Check sheet for the modelled part. Datum: model origin and axes. Units: mm. A direction names the side the tool comes from. Give positions to 0.01 mm unless a question says otherwise; leave off trailing zeros. Order: outer loops, then holes, each group sorted by start corner. A loop starts at its lowest first (then second) coordinate and runs counter-clockwise, first axis right, second up.
Item 1: Access from +Z, -Z, +X, -X, +Y, -Y to the whole of each face (thin tool, end or side, straight path). Record for faces 4 (the flat face through (0, 0, -14)), 5 (the flat face through (9.4, -2.9, 58.5)), 6 (the flat face through (0, -11.389, 62)), 7 (the flat face through (10, 0, 10)), 8 (the cylindrical face through (0, 14, 35)).
Item 2: Release check for a two-part mould opening along X. For faces 1 (the flat face through (0, -9, 59)), 2 (the cylindrical face through (3.233, 1.341, -0.986)), 3 (the cylindrical face through (11.5, 0.07, 4.93)) record: released by +X, released by -X, zero draft, split by the parting line, or undercut.
Item 3: Sectioned sample at A-A on z = 24. Record the boundary of the cut face in (x, y).
Item 4: Gauge pin test, flat ends, axial feed: P1, Ø1.5, axis at x = -9, y = -10, coming from the -Z side; P2, Ø4.5, axis at x = -2, y = -3.5, coming from the +Z side; P3, Ø1.5, axis at x = -10, y = 0, coming from the -Z side. Record the tip position at first contact, or that the pin passes through.
Item 5: Material ranges on line 1 along Z through (x, y) = (7.5, 6); line 2 along Y through (x, z) = (3.75, 42); line 3 along Z through (x, y) = (-10, -1), recorded low to high.
from build123d import *

# Parameters (mm, degrees)
SKETCH1_R            = 14
BOSS_EXTRUDE1_DEPTH  = 21
SKETCH2_R            = 13.5
BOSS_EXTRUDE2_DEPTH  = 0.5
SKETCH3_R            = 14
BOSS_EXTRUDE3_DEPTH  = 4
SKETCH4_R            = 14.5
BOSS_EXTRUDE4_DEPTH  = 20
SKETCH5_R            = 14
BOSS_EXTRUDE5_DEPTH  = 13
FILLET1_R            = 1
SKETCH6_R            = 14
SKETCH6_R_2          = 13.74791831
BOSS_EXTRUDE6_DEPTH  = 0.5
FILLET2_R            = 1
SKETCH7_R            = 5
BOSS_EXTRUDE7_DEPTH  = 3
SKETCH8_R            = 4.460837006
SKETCH8_R_2          = 1.021238478
CUT_EXTRUDE1_DEPTH   = 0.5
BOSS_EXTRUDE8_DEPTH  = 0.5
SKETCH10_W           = 3
SKETCH10_H           = 0.113026654
SKETCH10_H_2         = 0.277660136
BOSS_EXTRUDE9_DEPTH  = 6.5
FILLET3_R            = 0.4
CUT_EXTRUDE2_DEPTH   = 72.907798758
CUT_EXTRUDE3_DEPTH   = 0.1
CIRPATTERN1_COUNT    = 4
CUT_EXTRUDE4_DEPTH   = 45.949972191
SKETCH15_R           = 3.5
BOSS_EXTRUDE10_DEPTH = 2
SKETCH16_R           = 2
BOSS_EXTRUDE11_DEPTH = 12
CUT_EXTRUDE7_START   = -10
CUT_EXTRUDE7_DEPTH   = 10
SKETCH18_R           = 1.5
CUT_EXTRUDE8_DEPTH   = 10


with BuildPart() as part:
    # Sketch1 → Boss-Extrude1 (new body)
    with BuildSketch(Plane.XY):
        with Locations(Location((0, 0, 0), (0, 0, 180))):
            Circle(SKETCH1_R)
    extrude(amount=BOSS_EXTRUDE1_DEPTH)

    # Sketch2 → Boss-Extrude2 (add)
    with BuildSketch(Plane.XY.offset(21)):
        Circle(SKETCH2_R)
    extrude(amount=BOSS_EXTRUDE2_DEPTH)

    # Sketch3 → Boss-Extrude3 (add)
    with BuildSketch(Plane.XY.offset(21.5)):
        with Locations(Location((0, 0, 0), (0, 0, 180))):
            Circle(SKETCH3_R)
    extrude(amount=BOSS_EXTRUDE3_DEPTH)

    # Sketch4 → Boss-Extrude4 (add)
    with BuildSketch(Plane.XY.offset(25.5)):
        Circle(SKETCH4_R)
    extrude(amount=BOSS_EXTRUDE4_DEPTH)

    # Sketch5 → Boss-Extrude5 (add)
    with BuildSketch(Plane.XY.offset(45.5)):
        with Locations(Location((0, 0, 0), (0, 0, 180))):
            Circle(SKETCH5_R)
    extrude(amount=BOSS_EXTRUDE5_DEPTH)

    # Fillet1
    # the kernel refuses this fillet: 1 mm, written as the material it takes off along each edge
    with BuildSketch(Plane(origin=(0, 0, 21.5), x_dir=(-1, 0, 0), z_dir=(0, 1, 0))) as fillet1_piece_1:
        with BuildLine():
            CenterArc((13, 0.866025404), FILLET1_R, 300, 60)
            Line((13.5, 0), (13.51, -0.017320508))
            ThreePointArc((13.51, -0.017320508), (13.75, -0.02), (14, -0.02))
            Line((14, -0.02), (14.02, 0))
            Line((14.02, 0), (14.02, 0.866025404))
            Line((14.02, 0.866025404), (14, 0.866025404))
        make_face()
    revolve(axis=Axis((0, 0, 21.5), (0, 0, 1)), mode=Mode.SUBTRACT)

    # Sketch6 → Boss-Extrude6 (add)
    # profile 1 of 2: a face of its own
    with BuildSketch(Plane.XY.offset(58.5)):
        with Locations(Location((0, 0, 0), (0, 0, 180))):
            Circle(SKETCH6_R)
        Circle(SKETCH6_R_2, mode=Mode.SUBTRACT)
    # profile 2 of 2: a face of its own
    with BuildSketch(Plane.XY.offset(58.5)):
        with BuildLine():
            Line((-5, -8.077747211), (5, -8.077747211))
            ThreePointArc((5, -8.077747211), (9.5, 0), (5, 8.077747211))
            Line((5, 8.077747211), (-5, 8.077747211))
            ThreePointArc((-5, 8.077747211), (-9.5, 0), (-5, -8.077747211))
        make_face()
    extrude(amount=BOSS_EXTRUDE6_DEPTH)

    # Fillet2
    # the kernel refuses this fillet: 1 mm, written as the material it takes off along each edge
    with BuildSketch(Plane(origin=(0, 0, 59), x_dir=(-0.3204523861035329, 0.9472646241893299, 0), z_dir=(0.9472646241893299, 0.3204523861035329, 0))) as fillet2_piece_1:
        with BuildLine():
            CenterArc((8.633974596, -1), FILLET2_R, 30, 60)
            Line((9.5, -0.5), (9.517320508, -0.49))
            ThreePointArc((9.517320508, -0.49), (9.52, -0.25), (9.52, 0))
            Line((9.52, 0), (9.5, 0.02))
            Line((9.5, 0.02), (8.633974596, 0.02))
            Line((8.633974596, 0.02), (8.633974596, 0))
        make_face()
    revolve(axis=Axis((0, 0, 59), (0, 0, 1)), revolution_arc=142.619429044, mode=Mode.SUBTRACT)
    with BuildSketch(Plane(origin=(7.165063509, 8.077747211, 59), x_dir=(0, -1, 0), z_dir=(-1, 0, 0)), Plane(origin=(-7.165063509, -8.077747211, 59), x_dir=(0, 1, 0), z_dir=(1, 0, 0))) as fillet2_piece_2:
        with BuildLine():
            CenterArc((0.866025404, -1), FILLET2_R, 90, 60)
            Line((0, -0.5), (-0.017320508, -0.49))
            ThreePointArc((-0.017320508, -0.49), (-0.02, -0.25), (-0.02, 0))
            Line((-0.02, 0), (0, 0.02))
            Line((0, 0.02), (0.866025404, 0.02))
            Line((0.866025404, 0.02), (0.866025404, 0))
        make_face()
    extrude(amount=14.330127019, mode=Mode.SUBTRACT)
    with BuildSketch(Plane(origin=(0, 0, 59), x_dir=(0.3204523861035327, -0.9472646241893299, 0), z_dir=(-0.9472646241893299, -0.3204523861035327, 0))) as fillet2_piece_3:
        with BuildLine():
            CenterArc((8.633974596, -1), FILLET2_R, 30, 60)
            Line((8.633974596, 0), (8.633974596, 0.02))
            Line((8.633974596, 0.02), (9.5, 0.02))
            Line((9.5, 0.02), (9.52, 0))
            ThreePointArc((9.52, 0), (9.52, -0.25), (9.517320508, -0.49))
            Line((9.517320508, -0.49), (9.5, -0.5))
        make_face()
    revolve(axis=Axis((0, 0, 59), (0, 0, 1)), revolution_arc=142.619429044, mode=Mode.SUBTRACT)

    # Sketch7 → Boss-Extrude7 (add)
    with BuildSketch(Plane.XY.offset(59)):
        Circle(SKETCH7_R)
    extrude(amount=BOSS_EXTRUDE7_DEPTH)

    # Sketch8 → Cut-Extrude1 (cut)
    with BuildSketch(Plane.XY.offset(62)):
        Circle(SKETCH8_R)
        Circle(SKETCH8_R_2, mode=Mode.SUBTRACT)
    extrude(amount=-CUT_EXTRUDE1_DEPTH, mode=Mode.SUBTRACT)

    # Sketch9 → Boss-Extrude8 (add)
    with BuildSketch(Plane.XY.offset(58.5)):
        with BuildLine():
            Line((-4.864481732, 12.858540949), (-4.864481732, 8.474731605))
            Line((-4.864481732, 8.474731605), (3.898597634, 8.474731605))
            Line((3.898597634, 8.474731605), (3.898597634, 13.183557727))
            ThreePointArc((3.898597634, 13.183557727), (-0.509550782, 13.738472108), (-4.864481732, 12.858540949))
        make_face()
        with BuildLine():
            Line((-4.864481732, -12.858540949), (-4.864481732, -8.717904414))
            Line((-4.864481732, -8.717904414), (4.864481732, -8.717904414))
            Line((4.864481732, -8.717904414), (4.864481732, -12.858540949))
            ThreePointArc((4.864481732, -12.858540949), (0, -13.74791831), (-4.864481732, -12.858540949))
        make_face()
    extrude(amount=BOSS_EXTRUDE8_DEPTH)

    # Sketch10 → Boss-Extrude9 (add)
    with BuildSketch(Plane.XY.offset(59)):
        with Locations((0, 11.25)):
            Rectangle(SKETCH10_W, SKETCH10_H)
        with Locations((0, -11.25)):
            Rectangle(SKETCH10_W, SKETCH10_H_2)
    extrude(amount=BOSS_EXTRUDE9_DEPTH)

    # Fillet3
    fillet3_edges = [part.edges().sort_by_distance(p)[0] for p in [
        (1.5, 11.25, 65.5),
        (-1.5, 11.25, 65.5),
        (1.5, -11.25, 65.5),
        (-1.5, -11.25, 65.5),
    ]]
    fillet(fillet3_edges, radius=FILLET3_R)

    # Sketch11 → Cut-Extrude2 (cut, through all)
    with BuildSketch(Plane.XZ.offset(11.388830068)):
        with BuildLine():
            Line((0.372464769, 64.6226508), (0.372464769, 63.389034489))
            ThreePointArc((0.372464769, 63.389034489), (0, 63.016569721), (-0.372464769, 63.389034489))
            Line((-0.372464769, 63.389034489), (-0.372464769, 64.6226508))
            ThreePointArc((-0.372464769, 64.6226508), (0, 64.995115568), (0.372464769, 64.6226508))
        make_face()
    extrude(amount=-CUT_EXTRUDE2_DEPTH, mode=Mode.SUBTRACT)

    # Sketch12 → Cut-Extrude3 (cut)
    with BuildSketch(Plane(origin=(0, 0, 0), x_dir=(-1, 0, 0), z_dir=(0, 0, -1))):
        with BuildLine():
            Line((2.675792917, 7.20434815), (3.81405727, 10.269029513))
            ThreePointArc((3.81405727, 10.269029513), (4.376615733, 10.847932139), (5.183440496, 10.82275125))
            ThreePointArc((5.183440496, 10.82275125), (8.485281374, 8.485281374), (10.82275125, 5.183440496))
            ThreePointArc((10.82275125, 5.183440496), (10.847932139, 4.376615733), (10.269029513, 3.81405727))
            Line((10.269029513, 3.81405727), (7.20434815, 2.675792917))
            ThreePointArc((7.20434815, 2.675792917), (6.499150933, 2.679127181), (5.971506343, 3.147000475))
            ThreePointArc((5.971506343, 3.147000475), (4.772970773, 4.772970773), (3.147000475, 5.971506343))
            ThreePointArc((3.147000475, 5.971506343), (2.679127181, 6.499150933), (2.675792917, 7.20434815))
        make_face()
    cut_extrude3 = extrude(amount=-CUT_EXTRUDE3_DEPTH, mode=Mode.SUBTRACT)

    # CirPattern1: Cut-Extrude3 ×4 about axis
    cirpattern1_axis = Axis((0, 0, 0), (0, 0, 1))
    for i in range(1, CIRPATTERN1_COUNT):
        add(cut_extrude3.rotate(cirpattern1_axis, i * 360 / CIRPATTERN1_COUNT), mode=Mode.SUBTRACT)

    # Sketch13 → Cut-Extrude4 (cut, through all)
    with BuildSketch(Plane(origin=(0, 0, 25.5), x_dir=(-1, 0, 0), z_dir=(0, 0, -1))):
        with BuildLine():
            Line((-2.824925092, 13.712305557), (-3, 14.536259215))
            ThreePointArc((-3, 14.536259215), (0, 14.842601927), (3, 14.536259215))
            Line((3, 14.536259215), (2.824925092, 13.712305557))
            ThreePointArc((2.824925092, 13.712305557), (0, 14.000268764), (-2.824925092, 13.712305557))
        make_face()
    extrude(amount=-CUT_EXTRUDE4_DEPTH, mode=Mode.SUBTRACT)

    # Sketch15 → Boss-Extrude10 (add)
    with BuildSketch(Plane(origin=(0, 0, 0), x_dir=(-1, 0, 0), z_dir=(0, 0, -1))):
        with Locations(Location((0, 0, 0), (0, 0, 180))):
            Circle(SKETCH15_R)
    extrude(amount=BOSS_EXTRUDE10_DEPTH)

    # Sketch16 → Boss-Extrude11 (add)
    with BuildSketch(Plane(origin=(0, 0, -2), x_dir=(-1, 0, 0), z_dir=(0, 0, -1))):
        Circle(SKETCH16_R)
    extrude(amount=BOSS_EXTRUDE11_DEPTH)

    # Sketch17 → Cut-Extrude7 (cut)
    with BuildSketch(Plane(origin=(0, 0, -14), x_dir=(-1, 0, 0), z_dir=(0, 0, -1)).offset(CUT_EXTRUDE7_START)):
        with BuildLine():
            Line((-1.322875656, 1.5), (1.322875656, 1.5))
            ThreePointArc((1.322875656, 1.5), (0, 2), (-1.322875656, 1.5))
        make_face()
    extrude(amount=CUT_EXTRUDE7_DEPTH, mode=Mode.SUBTRACT)

    # Sketch18 → Cut-Extrude8 (cut)
    with BuildSketch(Plane(origin=(0, 0, 0), x_dir=(-1, 0, 0), z_dir=(0, 0, -1))):
        with Locations((-10, 0)):
            Circle(SKETCH18_R)
        with Locations((10, 0)):
            Circle(SKETCH18_R)
    extrude(amount=-CUT_EXTRUDE8_DEPTH, mode=Mode.SUBTRACT)


solid = part.part
Report:
1. face 4: -Z, +X, -X, +Y, -Y
1. face 5: +Z
1. face 6: +Z, +X, -X, -Y
1. face 7: -Z
1. face 8: +Z, -Z, +Y
2. face 1: zero draft
2. face 2: split by the parting line
2. face 3: undercut
3. outline: circle Ø28 at (0, 0)
4. P1: stops at z = 0
4. P2: stops at z = 62
4. P3: stops at z = 10
5. line 1: z = 0.1 to 58.5
5. line 2: y = -14.01 to 14.01
5. line 3: z = 10 to 58.5
